Design review of the part built by this model. Coordinates are the model's own, in mm. A direction names the side the tool comes from. Coordinates: 2 decimals unless noted, no trailing zeros. Loops run counter-clockwise (first coordinate to the right, second up) from the corner with the lowest first, then second, coordinate; pieces in that order, holes last. Notation, with made-up numbers: (73, 21.5) -> (103, 21.5) arc R14 cw to (103, 26.5) -> close; hole circle Ø11 at (-2, 39). An arc over 180 degrees is marked (long way). Use CSV: the item, a comma, the result in double quotes.
```python
from build123d import *

# Parameters (mm, degrees)
SKETCH3_W               = 40
SKETCH3_H               = 25
CUT_EXTRUDE1_DEPTH      = 290
CUT_EXTRUDE1_DEPTH_BACK = 290
SKETCH4_R               = 15
SKETCH5_W               = 110
SKETCH5_H               = 200
BOSS_EXTRUDE1_DEPTH     = 25
SKETCH6_W               = 94.303635564
SKETCH6_H               = 177.0699427
CUT_EXTRUDE2_DEPTH      = 5


with BuildPart() as part:
    # Sweep1: sweep along a path in Sketch2
    with BuildLine(Plane(origin=(0, 0, 0), x_dir=(0, 0, -1), z_dir=(1, 0, 0))) as sweep1_path:
        Line((-282.5, 0), (-282.5, 695))
        Line((-282.5, 695), (282.5, 695))
        Line((282.5, 695), (282.5, 0))
    # Sketch3 → Sweep1 (sweep)
    with BuildSketch(Plane(origin=(0, 0, 0), x_dir=(1, 0, 0), z_dir=(0, 1, 0))):
        with Locations((0, -282.5)):
            Rectangle(SKETCH3_W, SKETCH3_H)
    sweep(path=sweep1_path.line, transition=Transition.RIGHT)

    # Sketch4 → Cut-Extrude1 (cut, two sides: drawn at the far end of the back side and taken through both)
    with BuildSketch(Plane.XY.offset(-CUT_EXTRUDE1_DEPTH_BACK)):
        with Locations(Location((0, 25, 0), (0, 0, 180))):
            Circle(SKETCH4_R)
    extrude(amount=CUT_EXTRUDE1_DEPTH + CUT_EXTRUDE1_DEPTH_BACK, mode=Mode.SUBTRACT)

    # Sketch5 → Boss-Extrude1 (add)
    with BuildSketch(Plane(origin=(0, 707.5, 0), x_dir=(1, 0, 0), z_dir=(0, 1, 0))):
        Rectangle(SKETCH5_W, SKETCH5_H)
    extrude(amount=-BOSS_EXTRUDE1_DEPTH)

    # Sketch6 → Cut-Extrude2 (cut)
    with BuildSketch(Plane(origin=(0, 707.5, 0), x_dir=(1, 0, 0), z_dir=(0, 1, 0))):
        Rectangle(SKETCH6_W, SKETCH6_H)
    extrude(amount=-CUT_EXTRUDE2_DEPTH, mode=Mode.SUBTRACT)


solid = part.part
```
Item 1: To check wall thickness, follow line 1 along Z through (x, y) = (-17.5, 615); line 2 along Y through (x, z) = (0, -279); line 3 along Y through (x, z) = (42, -71). State the ranges of each line that lie inside material, in increasing order.
Checked values:
line 1,"-295 to -270, 270 to 295"
line 2,"0 to 10, 40 to 707.5"
line 3,"682.5 to 702.5"
Item 2: Machinability: for faces 1 (the face through (0, 346, 270)), 2 (the face through (3.252, 39.643, -280.14)), 3 (the face through (37, 695, 100)), 4 (the face through (-20, 407.8, -270.2)), 5 (the face through (37, 695, -100)), which of the approach directions +Z, -Z, +X, -X, +Y, -Y give a long, thin tool a straight path to every point of the face, cutting with its end or side? Answer none if there is none.
Checked values:
face 1,"+X, -X, -Y"
face 2,"none"
face 3,"+Z, +X, +Y, -Y"
face 4,"-Z, -X, +Y, -Y"
face 5,"-Z, +X, +Y, -Y"
Item 3: Add section A-A (y = 512). Give the boundary of the cut face in (x, z).
Checked values:
outline,"(-20, -295) -> (20, -295) -> (20, -270) -> (-20, -270) -> close; (-20, 270) -> (20, 270) -> (20, 295) -> (-20, 295) -> close"
Item 4: Draft analysis for pull direction Z (two halves, no side actions). For faces 6 (the face through (0, 336, -270)), 7 (the face through (3.252, 39.643, 279.86)), 8 (the face through (0, 349, -295)), 9 (the face through (20, 407.8, 270.2)), state which applies: pulls with the +Z half, pulls with the -Z half, needs draft (parallel to the pull), parting line crosses it, or undercut.
Checked values:
face 6,"undercut"
face 7,"undercut"
face 8,"pulls with the -Z half"
face 9,"needs draft"
Item 5: Add section B-B (x = 0). Give the boundary of the cut face in (y, z).
Checked values:
outline,"(0, -295) -> (707.5, -295) -> (707.5, -88.53) -> (702.5, -88.53) -> (702.5, 88.53) -> (707.5, 88.53) -> (707.5, 295) -> (0, 295) -> (0, 270) -> (10, 270) -> (10, 290) -> (40, 290) -> (40, 270) -> (682.5, 270) -> (682.5, -270) -> (40, -270) -> (40, -290) -> (10, -290) -> (10, -270) -> (0, -270) -> close"
Item 6: Clearance check with flat-ended pins moving along their axes: pin 1 (4 mm diameter, centred on x = -31.5, z = 65, fed in from -Y); pin 2 (7.5 mm diameter, centred on x = 31.5, y = 693, fed in from +Z). State where each tip first meets the part, or that it passes through.
Checked values:
pin 1,"y = 682.5"
pin 2,"z = 100"
Item 7: Add section D-D (y = 25). Give the boundary of the cut face in (x, z), then the cut area to 3 significant figures.
Checked values:
outline,"(-20, -295) -> (20, -295) -> (20, -270) -> (15, -270) -> (15, -290) -> (-15, -290) -> (-15, -270) -> (-20, -270) -> close; (-20, 270) -> (-15, 270) -> (-15, 290) -> (15, 290) -> (15, 270) -> (20, 270) -> (20, 295) -> (-20, 295) -> close"
area,"800 mm^2"
Item 8: Add section C-C (z = 78). Give the boundary of the cut face in (x, y).
Checked values:
outline,"(-55, 682.5) -> (55, 682.5) -> (55, 707.5) -> (47.15, 707.5) -> (47.15, 702.5) -> (-47.15, 702.5) -> (-47.15, 707.5) -> (-55, 707.5) -> close"
